CAD build for the part. Positions are in the model's coordinates, mm. Face numbers are marked on the shaded views. A direction names the side the tool comes from. Give positions to 0.01 mm unless a question says otherwise; leave off trailing zeros. Write each loop counter-clockwise with the first axis right and the second up, starting at its lowest first coordinate (ties: lowest second). Pieces come first, ordered by that corner, then holes. Notation, with made-up numbers: M -37,-8 L -30,-8 A32 cw -30,25 Z; hole C 63,-37 d7. An arc over 180 degrees is marked long. One line per question, with ' | ' between items. Start each with the question number.
1. Which spindle directions (+Z, -Z, +X, -X, +Y, -Y) get a long thin tool onto all of the face, cutting with end or side? Do the marked faces 5, 6, 7 and 8. Say none if no direction does.
2. Cut at C-C, the plane z = 4.5. Write the cut outline in (x, y).
3. Cut at B-B, the plane x = 13. Write the cut outline in (y, z), then the cut area to 3 significant figures.
4. Cut at D-D, the plane x = -3. Write the cut outline in (y, z).
5. Wall check: L1, parallel to X at y = 38, z = 7.5; L2, parallel to Y at x = 11, z = 2; L3, parallel to Y at x = 1.5, z = 6.25. Give the ranges that are in metal, low to high.
6. Pull direction Y, two halves, no side cores. Call the marked faces 1, 2, 3 and 4: released by +Y, released by -Y, zero draft, split by the parting line, or undercut.
7. Cut at A-A, the plane y = 43. Write the cut outline in (x, z), then the cut area to 3 significant figures.
8. Flat gauge pins, fed straight in: pin 1 (5 mm diameter, centred on x = 37.5, z = 7, fed in from +Y); pin 2 (2.5 mm diameter, centred on y = 16.5, z = 4.5, fed in from +X). Where does each tip first touch, or does it go through?
```python
from build123d import *

# Parameters (mm, degrees)
EXTRUDE_1_DEPTH = 10


with BuildPart() as part:
    # 草圖1 → 填料-伸長1 (new body)
    with BuildSketch(Plane.XY):
        with BuildLine():
            Line((7.459969379, 7.418851377), (61.73005582, 7.418851377))
            Line((61.73005582, 7.418851377), (61.73005582, 1.418851377))
            Line((61.73005582, 1.418851377), (-7.540030621, 1.418851377))
            Line((-7.540030621, 1.418851377), (-7.540030621, 22.324714328))
            Line((-7.540030621, 22.324714328), (-7.540030621, 32.418851377))
            Line((-7.540030621, 32.418851377), (5.553208045, 32.418851377))
            Line((5.553208045, 32.418851377), (5.553208045, 72.418851377))
            Line((5.553208045, 72.418851377), (20.553208045, 72.418851377))
            Line((20.553208045, 72.418851377), (20.553208045, 32.418851377))
            Line((20.553208045, 32.418851377), (43.60119499, 32.418851377))
            Line((43.60119499, 32.418851377), (43.60119499, 72.418851377))
            Line((43.60119499, 72.418851377), (58.60119499, 72.418851377))
            Line((58.60119499, 72.418851377), (58.60119499, 32.418851377))
            Line((58.60119499, 32.418851377), (61.73005582, 32.418851377))
            Line((61.73005582, 32.418851377), (61.73005582, 26.418851377))
            Line((61.73005582, 26.418851377), (7.459969379, 26.418851377))
            ThreePointArc((7.459969379, 26.418851377), (3.517633158, 24.620798228), (2.459969379, 20.418851377))
            Line((2.459969379, 20.418851377), (2.459969379, 12.418851377))
            ThreePointArc((2.459969379, 12.418851377), (3.924435473, 8.883317471), (7.459969379, 7.418851377))
        make_face()
    extrude(amount=EXTRUDE_1_DEPTH)


solid = part.part
```
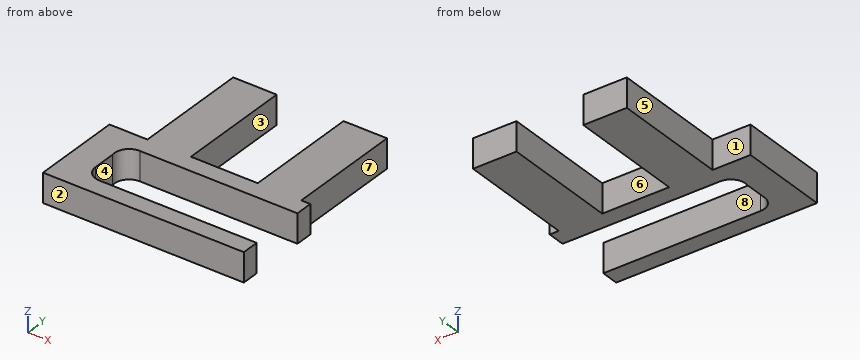
Here are the results:
1) face 5: +Z, -Z, -X, +Y | face 6: +Z, -Z, +Y | face 7: +Z, -Z, +X, +Y | face 8: +Z, -Z, +X
2) outline: M -7.54,1.42 L 61.73,1.42 L 61.73,7.42 L 7.46,7.42 A5 cw 2.46,12.42 L 2.46,20.42 A5 cw 7.46,26.42 L 61.73,26.42 L 61.73,32.42 L 58.6,32.42 L 58.6,72.42 L 43.6,72.42 L 43.6,32.42 L 20.55,32.42 L 20.55,72.42 L 5.55,72.42 L 5.55,32.42 L -7.54,32.42 Z
3) outline: M 1.42,0 L 7.42,0 L 7.42,10 L 1.42,10 Z; M 26.42,0 L 72.42,0 L 72.42,10 L 26.42,10 Z | area: 520 mm^2
4) outline: M 1.42,0 L 32.42,0 L 32.42,10 L 1.42,10 Z
5) L1: 5.55 to 20.55, 43.6 to 58.6 | L2: 1.42 to 7.42, 26.42 to 72.42 | L3: 1.42 to 32.42
6) face 1: released by +Y | face 2: released by -Y | face 3: zero draft | face 4: undercut
7) outline: M 5.55,0 L 20.55,0 L 20.55,10 L 5.55,10 Z; M 43.6,0 L 58.6,0 L 58.6,10 L 43.6,10 Z | area: 300 mm^2
8) pin 1: y = 32.42 | pin 2: x = 2.46
